Design review of the part built by this model. Coordinates are the model's own, in mm. A direction names the side the tool comes from. Give positions to 0.01 mm unless a question says otherwise; leave off trailing zeros. Order: outer loops, then holes, each group sorted by start corner. A loop starts at its lowest first (then second) coordinate and runs counter-clockwise, first axis right, second up. Notation, with made-up numbers: (57, -39) -> (69, -39) arc R25 ccw to (69, -7) -> close; hole circle Ø5 at (4.5, 71). An arc over 180 degrees is marked (long way). One line per item, written item: value.
from build123d import *

# Parameters (mm, degrees)
SKETCH1_R           = 2
BOSS_EXTRUDE1_DEPTH = 4
SKETCH2_W           = 25
SKETCH2_H           = 4
BOSS_EXTRUDE2_DEPTH = 12
SKETCH3_R           = 2
CUT_EXTRUDE1_DEPTH  = 12
FILLET1_R           = 2
FILLET2_R           = 1.5


with BuildPart() as part:
    # Sketch1 → Boss-Extrude1 (new body)
    with BuildSketch(Plane(origin=(0, 0, 0), x_dir=(1, 0, 0), z_dir=(0, 1, 0))):
        with BuildLine():
            Line((-4, 14.5), (21, 14.5))
            Line((21, 14.5), (21, -5))
            ThreePointArc((21, -5), (18.728627677, -8.607193695), (14.494076823, -8.117747429))
            ThreePointArc((14.494076823, -8.117747429), (7.866380142, -4.654307517), (0.418938394, -3.978000832))
            ThreePointArc((0.418938394, -3.978000832), (-2.676214343, -2.972856671), (-4, 0))
            Line((-4, 0), (-4, 14.5))
        make_face()
        with Locations(Location((0, 0, 0), (0, 0, 270))):
            Circle(SKETCH1_R, mode=Mode.SUBTRACT)
        with Locations(Location((17, -5, 0), (0, 0, 270))):
            Circle(SKETCH1_R, mode=Mode.SUBTRACT)
    extrude(amount=BOSS_EXTRUDE1_DEPTH)

    # Sketch2 → Boss-Extrude2 (add)
    with BuildSketch(Plane(origin=(0, 4, 0), x_dir=(1, 0, 0), z_dir=(0, 1, 0))):
        with Locations((8.5, 12.5)):
            Rectangle(SKETCH2_W, SKETCH2_H)
    extrude(amount=BOSS_EXTRUDE2_DEPTH)

    # Sketch3 → Cut-Extrude1 (cut)
    with BuildSketch(Plane.XY.offset(-10.5)):
        with Locations((2.25, 10)):
            Circle(SKETCH3_R)
        with Locations((14.75, 10)):
            Circle(SKETCH3_R)
    extrude(amount=-CUT_EXTRUDE1_DEPTH, mode=Mode.SUBTRACT)

    # Fillet1
    fillet1_edges = [part.edges().sort_by_distance(p)[0] for p in [
        (8.5, 4, -10.5),
    ]]
    fillet(fillet1_edges, radius=FILLET1_R)

    # Fillet2
    fillet2_edges = [part.edges().sort_by_distance(p)[0] for p in [
        (-2.676214343, 0, 2.972856671),
        (-4, 0, -7.25),
        (21, 0, -4.75),
        (18.728627677, 0, 8.607193695),
        (7.866380142, 0, 4.654307517),
    ]]
    fillet(fillet2_edges, radius=FILLET2_R)


solid = part.part
Item 1: Machinability: for faces 1 (the flat face through (8, 16, -13)), 2 (the flat face through (8, 11, -10.5)), which of the approach directions +Z, -Z, +X, -X, +Y, -Y give a long, thin tool a straight path to every point of the face, cutting with its end or side? Answer none if there is none.
Returned:
face 1: +Z, -Z, +X, -X, +Y
face 2: +Z, +X, -X, +Y
Item 2: Add section A-A on y = 10. Give the boundary of the cut face in (x, z), plus the area to 3 significant figures.
Returned:
outline: (-4, -14.5) -> (0.25, -14.5) -> (0.25, -10.5) -> (-4, -10.5) -> close; (4.25, -14.5) -> (12.75, -14.5) -> (12.75, -10.5) -> (4.25, -10.5) -> close; (16.75, -14.5) -> (21, -14.5) -> (21, -10.5) -> (16.75, -10.5) -> close
area: 68.0 mm²
Item 3: Add section C-C on y = 13.5. Give the boundary of the cut face in (x, z), plus the area to 3 significant figures.
Returned:
outline: (-4, -14.5) -> (21, -14.5) -> (21, -10.5) -> (-4, -10.5) -> close
area: 100 mm²
Item 4: Add section D-D on y = 2. Give the boundary of the cut face in (x, z), plus the area to 3 significant figures.
Returned:
outline: (-4, -14.5) -> (21, -14.5) -> (21, 5) arc R4 ccw to (14.49, 8.12) arc R19.25 cw to (0.42, 3.98) arc R4 ccw to (-4, 0) -> close; hole circle Ø4 at (0, 0); hole circle Ø4 at (17, 5)
area: 477 mm²
Item 5: Draft analysis for pull direction Z (two halves, no side actions). For faces 3 (the cylindrical face through (7.967, 2.732, 4.684)), 4 (the cylindrical face through (19, 2, 5)), 5 (the flat face through (9, 4, -2)), 6 (the flat face through (8, 8, -14.5)), state which applies: pulls with the +Z half, pulls with the -Z half, needs draft (parallel to the pull), parting line crosses it, or undercut.
Returned:
face 3: pulls with the +Z half
face 4: undercut
face 5: needs draft
face 6: pulls with the -Z half
Item 6: To check wall thickness, follow line 1 along Y through (x, z) = (14.75, -12.4); line 2 along X through (y, z) = (1.5, 0); line 3 along Z through (x, y) = (-1.5, 13). State the ranges of each line that lie inside material, in increasing order. Write a range as from..to.
Returned:
line 1: 0..8, 12..16
line 2: -4..-2, 2..21
line 3: -14.5..-10.5
Item 7: Clearance check with flat-ended pins moving along their axes: P1, Ø5, axis at x = 2.25, y = 10, coming from the +Z side; P2, Ø1.5, axis at y = 9.5, z = -10, coming from the +X side; P3, Ø8, axis at x = -1.5, z = 2.5, coming from the +Y side; P4, Ø6, axis at x = 5, y = 6.5, coming from the +Z side. State where each tip first meets the part, or that it passes through.
Returned:
P1: z = -10.5
P2: x = 21
P3: y = 4
P4: z = 4.34
Item 8: Add section B-B on z = -5.5. Give the boundary of the cut face in (x, y).
Returned:
outline: (-4, 1.5) arc R1.5 ccw to (-2.5, 0) -> (19.5, 0) arc R1.5 ccw to (21, 1.5) -> (21, 4) -> (-4, 4) -> close
